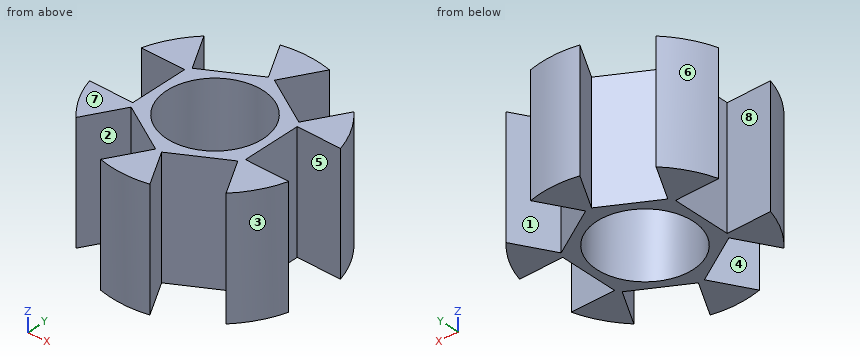
```python
from build123d import *

# Parameters (mm, degrees)
SKETCH1_R           = 8.75
SKETCH1_R_2         = 4.05
BOSS_EXTRUDE1_DEPTH = 5
SKETCH2_W           = 4.9
SKETCH2_H           = 10
CUT_EXTRUDE3_DEPTH  = 4
CIRPATTERN1_COUNT   = 6


with BuildPart() as part:
    # Sketch1 → Boss-Extrude1 (new body, symmetric)
    with BuildSketch(Plane.XY):
        Circle(SKETCH1_R)
        Circle(SKETCH1_R_2, mode=Mode.SUBTRACT)
    extrude(amount=BOSS_EXTRUDE1_DEPTH, both=True)

    # Sketch2 → Cut-Extrude3 (cut)
    with BuildSketch(Plane(origin=(-8.75, -17.193061184, 0), x_dir=(0, -1, 0), z_dir=(1, 0, 0))):
        with Locations((-17.193061184, 0)):
            Rectangle(SKETCH2_W, SKETCH2_H)
    cut_extrude3 = extrude(amount=CUT_EXTRUDE3_DEPTH, mode=Mode.SUBTRACT)

    # CirPattern1: Cut-Extrude3 ×6 about axis
    cirpattern1_axis = Axis((0, 0, 0), (0, 0, 1))
    for i in range(1, CIRPATTERN1_COUNT):
        add(cut_extrude3.rotate(cirpattern1_axis, i * 360 / CIRPATTERN1_COUNT), mode=Mode.SUBTRACT)


solid = part.part
```
Part model, mm, in its own coordinate system. Face numbers are marked on the shaded views. A direction names the side the tool comes from. Round coordinates to 2 decimals unless told otherwise and drop trailing zeros. Loops run counter-clockwise (first coordinate to the right, second up) from the corner with the lowest first, then second, coordinate; pieces in that order, holes last. Notation, with made-up numbers: (76.5, 68.5) -> (117.5, 68.5) arc R19 ccw to (117.5, 73.5) -> close; hole circle Ø11 at (77, 87). An arc over 180 degrees is marked (long way). Use one line per item in the form item = value. Start each with the question number.
Item 1: Tool access for the marked faces 1, 2, 3, 4 and 5: list every direction of +Z, -Z, +X, -X, +Y, -Y with a clear straight run to the whole face (end or side of a thin tool).
Item 2: Band-saw the part on D-D (y = -4.75). List the corners of the cut face in (x, z), plus the area to 3 significant figures.
Item 3: Band-saw the part on A-A (y = 0). List the corners of the cut face in (x, z).
Item 4: Drill centre lines: line 1 along X through (y, z) = (-5.75, -2.5); line 2 along Y through (x, z) = (0, -2.75); line 3 along X through (y, z) = (-3, -2.5). Where is each one in solid material? Low to high.
Item 5: Two-plate mould, pull along Y, no slides. Class the marked faces 6, 7 and 8: released by +Y, released by -Y, zero draft, split by the parting line, or undercut.
Item 6: Drop flat-ended pins along their axis: pin 1 Ø3 at (x, y) = (-4.5, -6.5) entering from -Z; pin 2 Ø4 at (y, z) = (-0.5, -1.5) entering from +X; pin 3 Ø1.8 at (x, z) = (6.5, 2.5) entering from +Y; pin 4 Ø1.1 at (x, z) = (-7.5, 1) entering from +Y. Give the stop position or say it passes through.
Item 7: Band-saw the part on C-C (z = 0.25). List the corners of the cut face in (x, y).
Item 8: Band-saw the part on B-B (x = 0). List the corners of the cut face in (y, z).
Data:
q1.face_1 = +Z, -Z, +Y
q1.face_2 = +Z, -Z, -Y
q1.face_3 = +Z, -Z, +X, -Y
q1.face_4 = +Z, -Z
q1.face_5 = +Z, -Z, +X
q2.outline = (-7.35, -5) -> (-5.57, -5) -> (-5.57, 5) -> (-7.35, 5) -> close; (-1.27, -5) -> (1.27, -5) -> (1.27, 5) -> (-1.27, 5) -> close; (5.57, -5) -> (7.35, -5) -> (7.35, 5) -> (5.57, 5) -> close
q2.area = 61.0 mm^2
q3.outline = (-4.75, -5) -> (-4.05, -5) -> (-4.05, 5) -> (-4.75, 5) -> close; (4.05, -5) -> (4.75, -5) -> (4.75, 5) -> (4.05, 5) -> close
q4.line_1 = -6.6 to -6.15, -0.49 to 0.49, 6.15 to 6.6
q4.line_2 = -8.75 to -4.05, 4.05 to 8.75
q4.line_3 = -8.22 to -4.56, -4.3 to -2.72, 2.72 to 4.3, 4.56 to 8.22
q5.face_6 = released by +Y
q5.face_7 = zero draft
q5.face_8 = undercut
q6.pin_1 = through
q6.pin_2 = 8.4
q6.pin_3 = 6.05
q6.pin_4 = 5.32
q7.outline = (-8.4, -2.45) arc R8.75 ccw to (-6.32, -6.05) -> (-4.5, -2.89) -> (-0.25, -5.34) -> (-2.08, -8.5) arc R8.75 ccw to (2.08, -8.5) -> (0.25, -5.34) -> (4.5, -2.89) -> (6.32, -6.05) arc R8.75 ccw to (8.4, -2.45) -> (4.75, -2.45) -> (4.75, 2.45) -> (8.4, 2.45) arc R8.75 ccw to (6.32, 6.05) -> (4.5, 2.89) -> (0.25, 5.34) -> (2.08, 8.5) arc R8.75 ccw to (-2.08, 8.5) -> (-0.25, 5.34) -> (-4.5, 2.89) -> (-6.32, 6.05) arc R8.75 ccw to (-8.4, 2.45) -> (-4.75, 2.45) -> (-4.75, -2.45) -> close; hole circle Ø8.1 at (0, 0)
q8.outline = (-8.75, -5) -> (-4.05, -5) -> (-4.05, 5) -> (-8.75, 5) -> close; (4.05, -5) -> (8.75, -5) -> (8.75, 5) -> (4.05, 5) -> close
